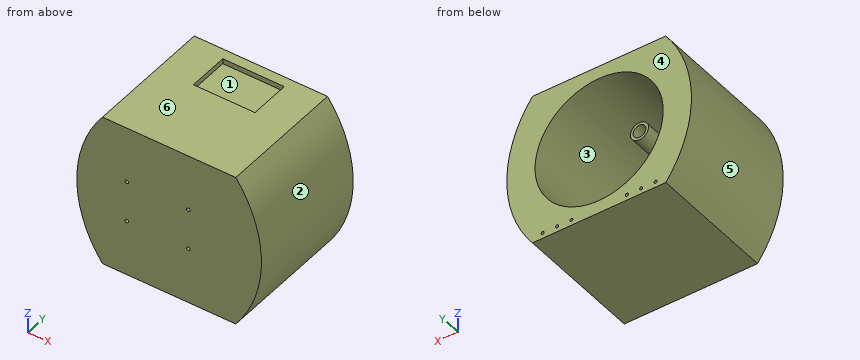
from build123d import *

# Parameters (mm, degrees)
BOSS_EXTRUDE1_DEPTH      = 250
INSIDE_COMPARTMENT_R     = 125
CUT_EXTRUDE1_DEPTH       = 240
LCD_W                    = 120
LCD_H                    = 80
CUT_EXTRUDE2_DEPTH       = 10
HINGE_HOLES_R            = 3
CUT_EXTRUDE3_DEPTH       = 20
POWER_SUPPLY_HOLES_R     = 3.5
CUT_EXTRUDE4_DEPTH       = 336.410196625
POLES_FOR_MIDDLE_LAYER_R = 17.5
BOSS_EXTRUDE2_DEPTH      = 130
HOLES_FOR_POLES_R        = 12.5
CUT_EXTRUDE6_DEPTH       = 50


with BuildPart() as part:
    # Case 2 → Boss-Extrude1 (new body)
    with BuildSketch(Plane(origin=(0, 0, 0), x_dir=(1, 0, 0), z_dir=(0, 1, 0))):
        with BuildLine():
            Line((-130, 150), (130, 150))
            ThreePointArc((130, 150), (180, 0), (130, -150))
            Line((130, -150), (-130, -150))
            ThreePointArc((-130, -150), (-180, 0), (-130, 150))
        make_face()
    extrude(amount=BOSS_EXTRUDE1_DEPTH)

    # Inside Compartment → Cut-Extrude1 (cut)
    with BuildSketch(Plane(origin=(0, 250, 0), x_dir=(1, 0, 0), z_dir=(0, 1, 0))):
        with Locations(Location((0, 0, 0), (0, 0, 270))):
            Circle(INSIDE_COMPARTMENT_R)
    extrude(amount=-CUT_EXTRUDE1_DEPTH, mode=Mode.SUBTRACT)

    # LCD → Cut-Extrude2 (cut)
    with BuildSketch(Plane.XY.offset(150)):
        with Locations((0, 190)):
            Rectangle(LCD_W, LCD_H)
    extrude(amount=-CUT_EXTRUDE2_DEPTH, mode=Mode.SUBTRACT)

    # Hinge holes → Cut-Extrude3 (cut)
    with BuildSketch(Plane(origin=(0, 250, 0), x_dir=(1, 0, 0), z_dir=(0, 1, 0))):
        with Locations(Location((-110, 139, 0), (0, 0, 270))):
            Circle(HINGE_HOLES_R)
        with Locations(Location((-82, 139, 0), (0, 0, 270))):
            Circle(HINGE_HOLES_R)
        with Locations(Location((-54, 139, 0), (0, 0, 270))):
            Circle(HINGE_HOLES_R)
        with Locations(Location((54, 139, 0), (0, 0, 270))):
            Circle(HINGE_HOLES_R)
        with Locations(Location((82, 139, 0), (0, 0, 270))):
            Circle(HINGE_HOLES_R)
        with Locations(Location((110, 139, 0), (0, 0, 270))):
            Circle(HINGE_HOLES_R)
    extrude(amount=-CUT_EXTRUDE3_DEPTH, mode=Mode.SUBTRACT)

    # Power supply holes → Cut-Extrude4 (cut, through all)
    with BuildSketch(Plane(origin=(0, 10, 0), x_dir=(1, 0, 0), z_dir=(0, 1, 0))):
        with Locations(Location((-82.5, 40, 0), (0, 0, 270))):
            Circle(POWER_SUPPLY_HOLES_R)
        with Locations(Location((37.5, 40, 0), (0, 0, 270))):
            Circle(POWER_SUPPLY_HOLES_R)
        with Locations(Location((37.5, -40, 0), (0, 0, 270))):
            Circle(POWER_SUPPLY_HOLES_R)
        with Locations(Location((-82.5, -40, 0), (0, 0, 270))):
            Circle(POWER_SUPPLY_HOLES_R)
    extrude(amount=-CUT_EXTRUDE4_DEPTH, mode=Mode.SUBTRACT)

    # Poles for middle layer → Boss-Extrude2 (add)
    with BuildSketch(Plane(origin=(0, 10, 0), x_dir=(1, 0, 0), z_dir=(0, 1, 0))):
        with Locations(Location((0, 90, 0), (0, 0, 270))):
            Circle(POLES_FOR_MIDDLE_LAYER_R)
        with Locations(Location((0, -90, 0), (0, 0, 270))):
            Circle(POLES_FOR_MIDDLE_LAYER_R)
    extrude(amount=BOSS_EXTRUDE2_DEPTH)

    # Holes for poles → Cut-Extrude6 (cut)
    with BuildSketch(Plane(origin=(0, 140, 0), x_dir=(1, 0, 0), z_dir=(0, 1, 0))):
        with Locations(Location((0, -90, 0), (0, 0, 270))):
            Circle(HOLES_FOR_POLES_R)
        with Locations(Location((0, 90, 0), (0, 0, 270))):
            Circle(HOLES_FOR_POLES_R)
    extrude(amount=-CUT_EXTRUDE6_DEPTH, mode=Mode.SUBTRACT)


solid = part.part
Read the model definition and answer for the solid it produces. Units are mm, in the model's axes. Face numbers are marked on the shaded views. A direction names the side the tool comes from. Give positions to 0.01 mm unless a question says otherwise; leave off trailing zeros. Write each loop counter-clockwise with the first axis right and the second up, starting at its lowest first coordinate (ties: lowest second). Pieces come first, ordered by that corner, then holes. Notation, with made-up numbers: (25.25, 22) - (45.25, 22) arc R30 cw to (45.25, 55) - close; hole circle Ø8 at (72, 16). An arc over 180 degrees is marked (long way). Answer in a Markdown table with one row per item. Add a question column.
Item 1: Section D-D, the plane z = -22 is taken. Write down the section's boundary in (x, y), and give its area (3 significant figures).
Item 2: Section A-A, the plane y = 97 is taken. Write down the section's boundary in (x, z).
Item 3: Flat-ended cylindrical pins translate along their axes: P1, Ø3, axis at y = 116.5, z = 100.5, coming from the +X side; P2, Ø5, axis at x = 81.5, z = -139.5, coming from the +Y side; P3, Ø8, axis at y = 201, z = 143, coming from the +X side; P4, Ø10.5, axis at x = -4.5, z = 86.5, coming from the +Y side. Find the tip coordinate at first contact, or state that the pin passes through.
Item 4: A tool of negligible diameter and unlimited length cuts with its end or side. For the marked faces 1 and 2, from which of +Z, -Z, +X, -X, +Y, -Y can it reach the whole face along a straight path? Write none if from no direction.
Item 5: Find the intervals of material crossed by L1, parallel to Z at x = -1.5, y = 46; L2, parallel to Z at x = 0.5, y = 222; L3, parallel to X at y = 3.5, z = 40, in increasing order.
Item 6: Section C-C, the plane x = 0 is taken. Write down the section's boundary in (y, z), and give its area (3 significant figures).
Item 7: Determine the mould class of the marked faces 3, 4, 5 and 6 for opening direction Z: pulls with the +Z half, pulls with the -Z half, needs draft (parallel to the pull), parting line crosses it, or undercut.
Item 8: Section B-B, the plane y = 36 is taken. Write down the section's boundary in (x, z).
Recorded:
| question | item | result |
|---|---|---|
| 1 | outline | (-179.03, 0) - (179.03, 0) - (179.03, 250) - (123.05, 250) - (123.05, 10) - (-123.05, 10) - (-123.05, 250) - (-179.03, 250) - close |
| 1 | area | 30,500 mm2 |
| 2 | outline | (-130, -150) - (130, -150) arc R250 ccw to (130, 150) - (-130, 150) arc R250 ccw to start; circle Ø35 at (0, -90); circle Ø35 at (0, 90); hole circle Ø250 at (0, 0); hole circle Ø25 at (0, -90); hole circle Ø25 at (0, 90) |
| 3 | P1 | stops at x = 159.56 |
| 3 | P2 | stops at y = 250 |
| 3 | P3 | stops at x = 137.8 |
| 3 | P4 | stops at y = 90 |
| 4 | face 1 | +Z |
| 4 | face 2 | +X, +Y, -Y |
| 5 | L1 | z = -150 to -124.99, -107.44 to -72.56, 72.56 to 107.44, 124.99 to 150 |
| 5 | L2 | z = -150 to -125, 125 to 140 |
| 5 | L3 | x = -176.78 to -86, -79 to 34, 41 to 176.78 |
| 6 | outline | (0, -150) - (250, -150) - (250, -125) - (10, -125) - (10, -107.5) - (140, -107.5) - (140, -102.5) - (90, -102.5) - (90, -77.5) - (140, -77.5) - (140, -72.5) - (10, -72.5) - (10, 72.5) - (140, 72.5) - (140, 77.5) - (90, 77.5) - (90, 102.5) - (140, 102.5) - (140, 107.5) - (10, 107.5) - (10, 125) - (250, 125) - (250, 150) - (230, 150) - (230, 140) - (150, 140) - (150, 150) - (0, 150) - close |
| 6 | area | 20,800 mm2 |
| 7 | face 3 | undercut |
| 7 | face 4 | needs draft |
| 7 | face 5 | parting line crosses it |
| 7 | face 6 | pulls with the +Z half |
| 8 | outline | (-130, -150) - (130, -150) arc R250 ccw to (130, 150) - (-130, 150) arc R250 ccw to start; circle Ø35 at (0, -90); circle Ø35 at (0, 90); hole circle Ø250 at (0, 0) |
